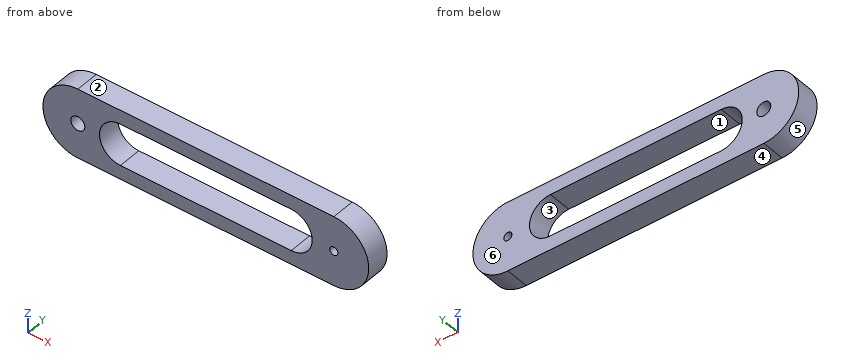
```python
from build123d import *

# Parameters (mm, degrees)
SKETCH2_R           = 1.45
SKETCH2_R_2         = 1.5
BOSS_EXTRUDE1_DEPTH = 10
SKETCH3_R           = 2.925
CUT_EXTRUDE1_DEPTH  = 2
CUT_EXTRUDE2_DEPTH  = 10
SKETCH5_R           = 3
CUT_EXTRUDE3_DEPTH  = 10
SKETCH6_R           = 1.75
CUT_EXTRUDE4_DEPTH  = 10


with BuildPart() as part:
    # Sketch2 → Boss-Extrude1 (new body)
    with BuildSketch(Plane(origin=(0, 0, 0), x_dir=(1, 0, 0), z_dir=(0, 1, 0))):
        with BuildLine():
            Line((0, 15), (110, 15))
            ThreePointArc((110, 15), (125, 0), (110, -15))
            Line((110, -15), (0, -15))
            ThreePointArc((0, -15), (-15, 0), (0, 15))
        make_face()
        with Locations(Location((0, 0, 0), (0, 0, 270))):
            Circle(SKETCH2_R, mode=Mode.SUBTRACT)
        with Locations(Location((110, 0, 0), (0, 0, 270))):
            Circle(SKETCH2_R_2, mode=Mode.SUBTRACT)
    extrude(amount=BOSS_EXTRUDE1_DEPTH)

    # Sketch3 → Cut-Extrude1 (cut)
    with BuildSketch(Plane(origin=(0, 10, 0), x_dir=(1, 0, 0), z_dir=(0, 1, 0))):
        with Locations(Location((0, 0, 0), (0, 0, 270))):
            Circle(SKETCH3_R)
    extrude(amount=-CUT_EXTRUDE1_DEPTH, mode=Mode.SUBTRACT)

    # Sketch4 → Cut-Extrude2 (cut)
    with BuildSketch(Plane(origin=(0, 10, 0), x_dir=(1, 0, 0), z_dir=(0, 1, 0))):
        with BuildLine():
            Line((18.295710574, 9), (91.7, 9))
            ThreePointArc((91.7, 9), (100.7, 0), (91.7, -9))
            Line((91.7, -9), (18.295710574, -9))
            ThreePointArc((18.295710574, -9), (9.295710574, 0), (18.295710574, 9))
        make_face()
    extrude(amount=-CUT_EXTRUDE2_DEPTH, mode=Mode.SUBTRACT)

    # Sketch5 → Cut-Extrude3 (cut)
    with BuildSketch(Plane(origin=(0, 10, 0), x_dir=(1, 0, 0), z_dir=(0, 1, 0))):
        with Locations(Location((0, 0, 0), (0, 0, 270))):
            Circle(SKETCH5_R)
    extrude(amount=-CUT_EXTRUDE3_DEPTH, mode=Mode.SUBTRACT)

    # Sketch6 → Cut-Extrude4 (cut)
    with BuildSketch(Plane(origin=(0, 10, 0), x_dir=(1, 0, 0), z_dir=(0, 1, 0))):
        with Locations(Location((110, 0, 0), (0, 0, 270))):
            Circle(SKETCH6_R)
    extrude(amount=-CUT_EXTRUDE4_DEPTH, mode=Mode.SUBTRACT)


solid = part.part
```
CAD build for the part. Positions are in the model's coordinates, mm. Face numbers are marked on the shaded views. A direction names the side the tool comes from. Round coordinates to 2 decimals unless told otherwise and drop trailing zeros. Write each loop counter-clockwise with the first axis right and the second up, starting at its lowest first coordinate (ties: lowest second). Pieces come first, ordered by that corner, then holes. Notation, with made-up numbers: (-30.75, 26) - (-4.75, 26) arc R31 cw to (-4.75, 59) - close; hole circle Ø8 at (64, 24). An arc over 180 degrees is marked (long way). Return JSON: item names as keys, results as strings. Group by question number.
Item 1: Band-saw the part on C-C on z = -7.5. List the corners of the cut face in (x, y), plus the area to 3 significant figures.
Item 2: Band-saw the part on A-A on z = 0. List the corners of the cut face in (x, y).
Item 3: Band-saw the part on B-B on y = 2.25. List the corners of the cut face in (x, z), plus the area to 3 significant figures.
Item 4: Flat gauge pins, fed straight in: pin 1 Ø3 at (y, z) = (4.5, 11) entering from -X; pin 2 Ø4 at (x, z) = (110, 0) entering from -Y; pin 3 Ø3.5 at (x, z) = (0, 0) entering from -Y; pin 4 Ø3 at (y, z) = (6.5, 5) entering from -X. Where does each tip first touch, or does it go through?
Item 5: Mould opens along Z. For the marked faces 3, 4, 5 and 6 say: +Z half, -Z half, draft (parallel to the pull), parting line (faces both ways), or undercut.
Item 6: 3-axis set-ups, long thin cutter, end or side, ignore diameter. For the marked faces 1 and 2: which of +Z, -Z, +X, -X, +Y, -Y reach the whole face in a straight line?
Item 7: Probe probe 1 along X at (y, z) = (5, 0); probe 2 along Z at (x, y) = (85.5, 5.5); probe 3 along Z at (x, y) = (110, 4.5). List the from-to ranges inside material, lowest first.
Resolved:
{
 "1": {"outline": "(-12.99, 0) - (13.32, 0) - (13.32, 10) - (-12.99, 10) - close; (96.67, 0) - (122.99, 0) - (122.99, 10) - (96.67, 10) - close", "area": "526 mm²"},
 "2": {"outline": "(-15, 0) - (-3, 0) - (-3, 10) - (-15, 10) - close; (3, 0) - (9.3, 0) - (9.3, 10) - (3, 10) - close; (100.7, 0) - (108.25, 0) - (108.25, 10) - (100.7, 10) - close; (111.75, 0) - (125, 0) - (125, 10) - (111.75, 10) - close"},
 "3": {"outline": "(0, -15) - (110, -15) arc R15 ccw to (110, 15) - (0, 15) arc R15 ccw to start; hole circle Ø6 at (0, 0); hole (18.3, -9) - (91.7, -9) arc R9 ccw to (91.7, 9) - (18.3, 9) arc R9 ccw to start; hole circle Ø3.5 at (110, 0)", "area": "2,390 mm²"},
 "4": {"pin 1": "stops at x = -11.61", "pin 2": "stops at y = 0", "pin 3": "passes through", "pin 4": "stops at x = -14.59"},
 "5": {"face 3": "undercut", "face 4": "-Z half", "face 5": "parting line", "face 6": "draft"},
 "6": {"face 1": "+Y, -Y", "face 2": "+Z, +X, -X, +Y, -Y"},
 "7": {"probe 1": "x = -15 to -3, 3 to 9.3, 100.7 to 108.25, 111.75 to 125", "probe 2": "z = -15 to -9, 9 to 15", "probe 3": "z = -15 to -1.75, 1.75 to 15"}
}
